```python
from build123d import *

# Parameters (mm, degrees)
F3_R      = 4.7
F4_DEPTH  = 92
F8_DEPTH  = 92
F6_R      = 4.7
F6_R_2    = 4
F9_DEPTH  = 10
F7_R      = 4.7
F7_R_2    = 4
F10_DEPTH = 12
F11_R     = 2.75
F12_DEPTH = 4.701


# Not quite as in the source:
# - ends of sketch curves that miss each other by under 0.0002 mm in the source are joined


with BuildPart() as f4:
    # F3 (on Front) → F4 (new body)
    with BuildSketch(Plane.XZ):
        Circle(F3_R)
    extrude(amount=F4_DEPTH)

    # F5 (on face) → F8 (cut, through all)
    with BuildSketch(Plane.XZ.offset(92)):
        with BuildLine():
            Line((-1.25, -3.8), (0, -3.8))
            Line((0, -3.8), (1.25, -3.8))
            Line((1.25, -3.8), (1.25, -3.7))
            ThreePointArc((1.25, -3.7), (1.3085786438, -3.5585786438), (1.45, -3.5))
            Line((1.45, -3.5), (2, -3.5))
            Line((2, -3.5), (2, -3.05))
            ThreePointArc((2, -3.05), (2.0585786438, -2.9085786438), (2.2, -2.85))
            Line((2.2, -2.85), (3.15, -2.85))
            Line((3.15, -2.85), (3.15, -2.15))
            Line((3.15, -2.15), (2.2, -2.15))
            ThreePointArc((2.2, -2.15), (2.0585786438, -2.0914213562), (2, -1.95))
            Line((2, -1.95), (2, -1.887459))
            ThreePointArc((2, -1.887459), (2.1033535752, -1.771554046), (2.2, -1.65))
            Line((2.2, -1.65), (3.75, -1.65))
            Line((3.75, -1.65), (3.75, 0))
            Line((3.75, 0), (3.75, 1.65))
            Line((3.75, 1.65), (2.2, 1.65))
            ThreePointArc((2.2, 1.65), (2.1033535752, 1.771554046), (1.9999998047, 1.8874588157))
            Line((1.9999998047, 1.8874588157), (2, 1.95))
            ThreePointArc((2, 1.95), (2.0585786438, 2.0914213562), (2.2, 2.15))
            Line((2.2, 2.15), (3.15, 2.15))
            Line((3.15, 2.15), (3.15, 2.85))
            Line((3.15, 2.85), (2.2, 2.85))
            ThreePointArc((2.2, 2.85), (2.0585786438, 2.9085786438), (2, 3.05))
            Line((2, 3.05), (2, 3.5))
            Line((2, 3.5), (1.45, 3.5))
            ThreePointArc((1.45, 3.5), (1.3085786438, 3.5585786438), (1.25, 3.7))
            Line((1.25, 3.7), (1.25, 3.8))
            Line((1.25, 3.8), (0, 3.8))
            Line((0, 3.8), (-1.25, 3.8))
            Line((-1.25, 3.8), (-1.25, 3.7))
            ThreePointArc((-1.25, 3.7), (-1.3085786438, 3.5585786438), (-1.45, 3.5))
            Line((-1.45, 3.5), (-2, 3.5))
            Line((-2, 3.5), (-2, 3.05))
            ThreePointArc((-2, 3.05), (-2.0585786438, 2.9085786438), (-2.2, 2.85))
            Line((-2.2, 2.85), (-3.15, 2.85))
            Line((-3.15, 2.85), (-3.15, 2.15))
            Line((-3.15, 2.15), (-2.2, 2.15))
            ThreePointArc((-2.2, 2.15), (-2.0585786438, 2.0914213562), (-2, 1.95))
            Line((-2, 1.95), (-2, 1.887459))
            ThreePointArc((-2, 1.887459), (-2.1033535752, 1.771554046), (-2.2, 1.65))
            Line((-2.2, 1.65), (-3.75, 1.65))
            Line((-3.75, 1.65), (-3.75, 0))
            Line((-3.75, 0), (-3.75, -1.65))
            Line((-3.75, -1.65), (-2.2, -1.65))
            ThreePointArc((-2.2, -1.65), (-2.1033535752, -1.771554046), (-1.9999998047, -1.8874588157))
            Line((-1.9999998047, -1.8874588157), (-2, -1.95))
            ThreePointArc((-2, -1.95), (-2.0585786438, -2.0914213562), (-2.2, -2.15))
            Line((-2.2, -2.15), (-3.15, -2.15))
            Line((-3.15, -2.15), (-3.15, -2.85))
            Line((-3.15, -2.85), (-2.2, -2.85))
            ThreePointArc((-2.2, -2.85), (-2.0585786438, -2.9085786438), (-2, -3.05))
            Line((-2, -3.05), (-2, -3.5))
            Line((-2, -3.5), (-1.45, -3.5))
            ThreePointArc((-1.45, -3.5), (-1.3085786438, -3.5585786438), (-1.25, -3.7))
            Line((-1.25, -3.7), (-1.25, -3.8))
        make_face()
    extrude(amount=-F8_DEPTH, mode=Mode.SUBTRACT)

    # F6 (on face) → F9 (join)
    with BuildSketch(Plane.XZ.offset(92)):
        Circle(F6_R)
        Circle(F6_R_2, mode=Mode.SUBTRACT)
    extrude(amount=F9_DEPTH)

    # F7 (on face) → F10 (join)
    with BuildSketch(Plane(origin=(0, 0, 0), x_dir=(-1, 0, 0), z_dir=(0, 1, 0))):
        Circle(F7_R)
        Circle(F7_R_2, mode=Mode.SUBTRACT)
    extrude(amount=F10_DEPTH)

    # F11 (on Right) → F12 (cut, through all)
    with BuildSketch(Plane.YZ):
        with Locations((-95.75, 0)):
            Circle(F11_R)
    extrude(amount=-F12_DEPTH, mode=Mode.SUBTRACT)


solid = f4.part
```
Read the model definition and answer for the solid it produces. Units are mm, in the model's axes. A direction names the side the tool comes from. Give positions to 0.01 mm unless a question says otherwise; leave off trailing zeros. Order: outer loops, then holes, each group sorted by start corner. A loop starts at its lowest first (then second) coordinate and runs counter-clockwise, first axis right, second up.
(1) For faces 1 (the flat face through (0, -47, 3.8)), 2 (the cylindrical face through (0.867, 5.916, -3.905)), 3 (the cylindrical face through (-4.19, -93.13, 0.83)), 4 (the cylindrical face through (3.815, -96.93, 1.201)), determine the directions among +Z, -Z, +X, -X, +Y, -Y from which every point of the face is accessible in a straight line to the end or side of a thin tool.
(2) Find section C-C (y = -95.75). Give the vertices of the cut face in (x, z).
(3) For a pull along X with two mould halves and no side action, classify faces 5 (the flat face through (-3.75, -47, 0)), 6 (the flat face through (2, -102, 4)) as released by +X, released by -X, zero draft, split by the parting line, or undercut.
(4) Given pin 1 (2 mm diameter, centred on y = -74, z = -1.5, fed in from -X); pin 2 (0.5 mm diameter, centred on y = -43, z = 3.5, fed in from +X); pin 3 (0.8 mm diameter, centred on x = -2.5, y = -33, fed in from +Z), each flat-ended and moving along its own axis, determine where each tip first touches the part or whether it passes through.
(5) Find section B-B (z = 0). Give the vertices of the cut face in (x, y).
(6) Straight lines are drawn through the part: L1, parallel to Z at x = 0, y = -94.25; L2, parallel to Z at x = 0.25, y = -8.5; L3, parallel to Z at x = -3, y = -9. For each, find the intervals that lie inside material, in ascending order.
(7) Find section A-A (x = 0). Give the vertices of the cut face in (y, z).
Result sheet:
1. face 1: +Y, -Y
1. face 2: +Y
1. face 3: -X
1. face 4: -Y
2. outline: (-3.81, -2.75) arc R4.7 ccw (long way) to (-3.81, 2.75) - (-2.9, 2.75) arc R4 cw (long way) to (-2.9, -2.75) - close
3. face 5: undercut
3. face 6: zero draft
4. pin 1: stops at x = -4.67
4. pin 2: stops at x = 3.4
4. pin 3: stops at z = 4.2
5. outline: (-4.7, -102) - (-4, -102) - (-4, -98.5) - (-4.7, -98.5) - close; (-4.7, -93) - (-4, -93) - (-4, -92) - (-3.75, -92) - (-3.75, 0) - (-4, 0) - (-4, 12) - (-4.7, 12) - close; (3.75, -92) - (4, -92) - (4, -102) - (4.7, -102) - (4.7, 12) - (4, 12) - (4, 0) - (3.75, 0) - close
6. L1: z = -4.7 to -4, 4 to 4.7
6. L2: z = -4.69 to -3.8, 3.8 to 4.69
6. L3: z = -3.62 to -2.85, -2.15 to -1.65, 1.65 to 2.15, 2.85 to 3.62
7. outline: (-102, -4.7) - (12, -4.7) - (12, -4) - (0, -4) - (0, -3.8) - (-92, -3.8) - (-92, -4) - (-102, -4) - close; (-102, 4) - (-92, 4) - (-92, 3.8) - (0, 3.8) - (0, 4) - (12, 4) - (12, 4.7) - (-102, 4.7) - close
